Check sheet for the drawn part. Datum: minimum x, y, z corner. Units: mm. Round coordinates to 2 decimals unless told otherwise and drop trailing zeros. Order: outer loops, then holes, each group sorted by start corner. A loop starts at its lowest first (then second) coordinate and runs counter-clockwise, first axis right, second up. Notation, with made-up numbers: (37, 76) -> (68, 76) arc R23 cw to (68, 85) -> close; hole circle Ø9 at (-0.75, 55.5). An arc over 180 degrees is marked (long way). Answer as a JSON object with one key per item and string values. Group by question number.
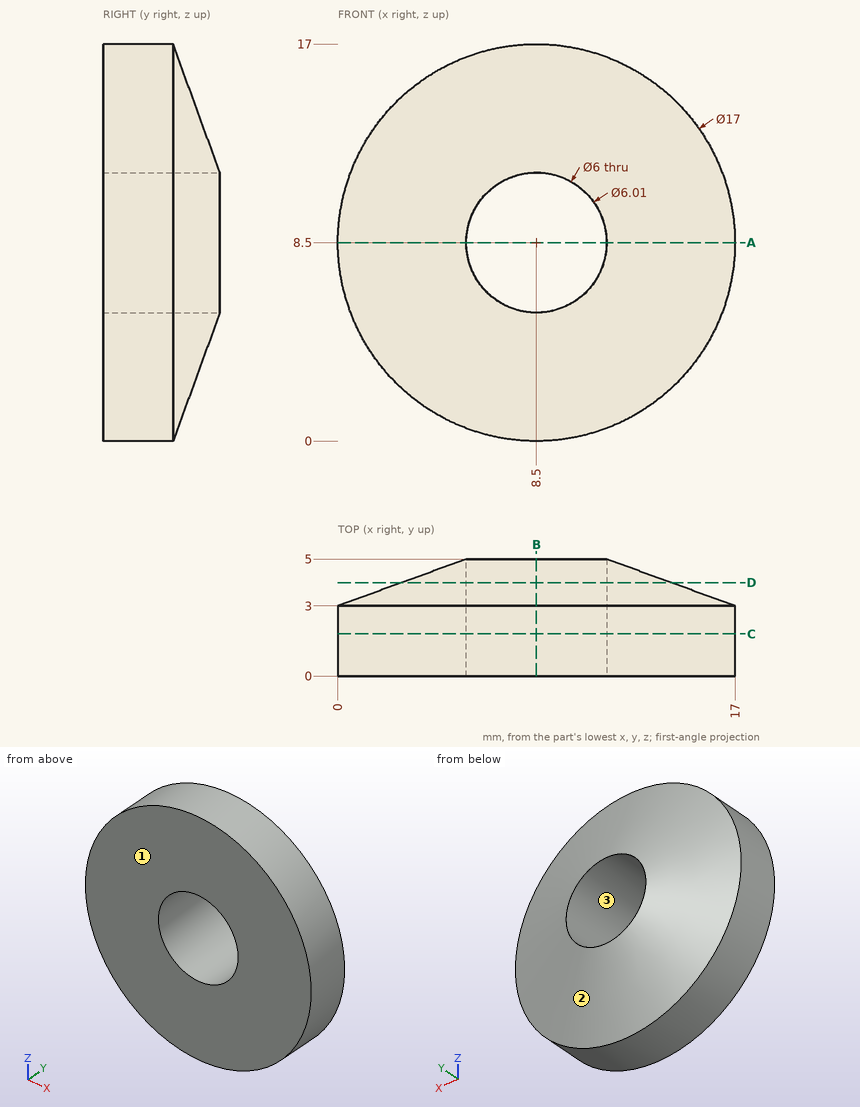
Item 1: Sectioned sample at D-D, the plane y = 4. Enter the section's corners in (x, z) (1 decimal), then the cut area to 3 significant figures.
Item 2: Depth check by flat-ended pin: pin 1 Ø1 at (x, z) = (4.5, 11.5) entering from +Y; pin 2 Ø2 at (y, z) = (3.5, 8.5) entering from +X; pin 3 Ø3 at (x, z) = (14.5, 13.5) entering from +Y. Enter the tip coordinate at first touch or a pass-through.
Item 3: Sectioned sample at A-A, the plane z = 8.5. Enter the section's corners in (x, y) (3 decimals), then the cut area to 3 significant figures.
Item 4: Mould release check, pull along X, two halves, no side actions. Record for the marked faces 1, 2 and 3: pulls with the +X half, pulls with the -X half, needs draft (parallel to the pull), parting line crosses it, or undercut.
Item 5: Sectioned sample at C-C, the plane y = 1.8. Enter the section's corners in (x, z), then the cut area to 3 significant figures.
Item 6: Thickness scan on L1, parallel to Z at x = 8.5, y = 2.3; L2, parallel to Z at x = 7.5, y = 1.4. Record the ranges inside material, lowest first.
Item 7: Sectioned sample at B-B, the plane x = 8.5. Enter the section's corners in (y, z) (3 decimals).
Result:
{
 "1": {"outline": "circle Ø11.5 at (8.5, 8.5); hole circle Ø6 at (8.5, 8.5)", "area": "75.7 mm2"},
 "2": {"pin 1": "stops at y = 4.46", "pin 2": "stops at x = 17", "pin 3": "stops at y = 3.8"},
 "3": {"outline": "(0, 0) -> (5.5, 0) -> (5.5, 5) -> (5.495, 5) -> (0, 3) -> close; (11.5, 0) -> (17, 0) -> (17, 3) -> (11.505, 5) -> (11.5, 5) -> close", "area": "44.0 mm2"},
 "4": {"face 1": "needs draft", "face 2": "parting line crosses it", "face 3": "undercut"},
 "5": {"outline": "circle Ø17 at (8.5, 8.5); hole circle Ø6 at (8.5, 8.5)", "area": "199 mm2"},
 "6": {"L1": "z = 0 to 5.5, 11.5 to 17", "L2": "z = 0.06 to 5.67, 11.33 to 16.94"},
 "7": {"outline": "(0, 0) -> (3, 0) -> (5, 5.495) -> (5, 5.5) -> (0, 5.5) -> close; (0, 11.5) -> (5, 11.5) -> (5, 11.505) -> (3, 17) -> (0, 17) -> close"}
}
